Check sheet for the drawn part. Datum: minimum x, y, z corner. Units: mm. Round coordinates to 2 decimals unless told otherwise and drop trailing zeros. Write each loop counter-clockwise with the first axis right and the second up, starting at its lowest first coordinate (ties: lowest second). Pieces come first, ordered by that corner, then holes. Notation, with made-up numbers: (-25.75, 63) - (30.25, 63) arc R11 ccw to (30.25, 73) - close; hole circle Ø8 at (-28, 87). An arc over 180 degrees is marked (long way). Answer as a JSON object with one key per item and string values. Group by question number.
Item 1: Gauge pin test, flat end, axial feed: P1, Ø1.5, axis at y = 1.5, z = 1, coming from the -X side. Record the tip position at first contact, or that the pin passes through.
Item 2: Sectioned sample at A-A on x = 7. Record the boundary of the cut face in (y, z), plus the area to 3 significant figures.
Item 3: Release check for a two-part mould opening along Y. For the marked faces 1, 2 and 3 record: pulls with the +Y half, pulls with the -Y half, needs draft (parallel to the pull), parting line crosses it, or undercut.
Item 4: Sectioned sample at C-C on z = 9.25. Record the boundary of the cut face in (x, y), plus the area to 3 significant figures.
Item 5: Thickness scan on line 1 (Y direction, x = 7, z = 7.25); line 2 (Y direction, x = 4.75, z = 1.25). Record the ranges inside material, lowest first.
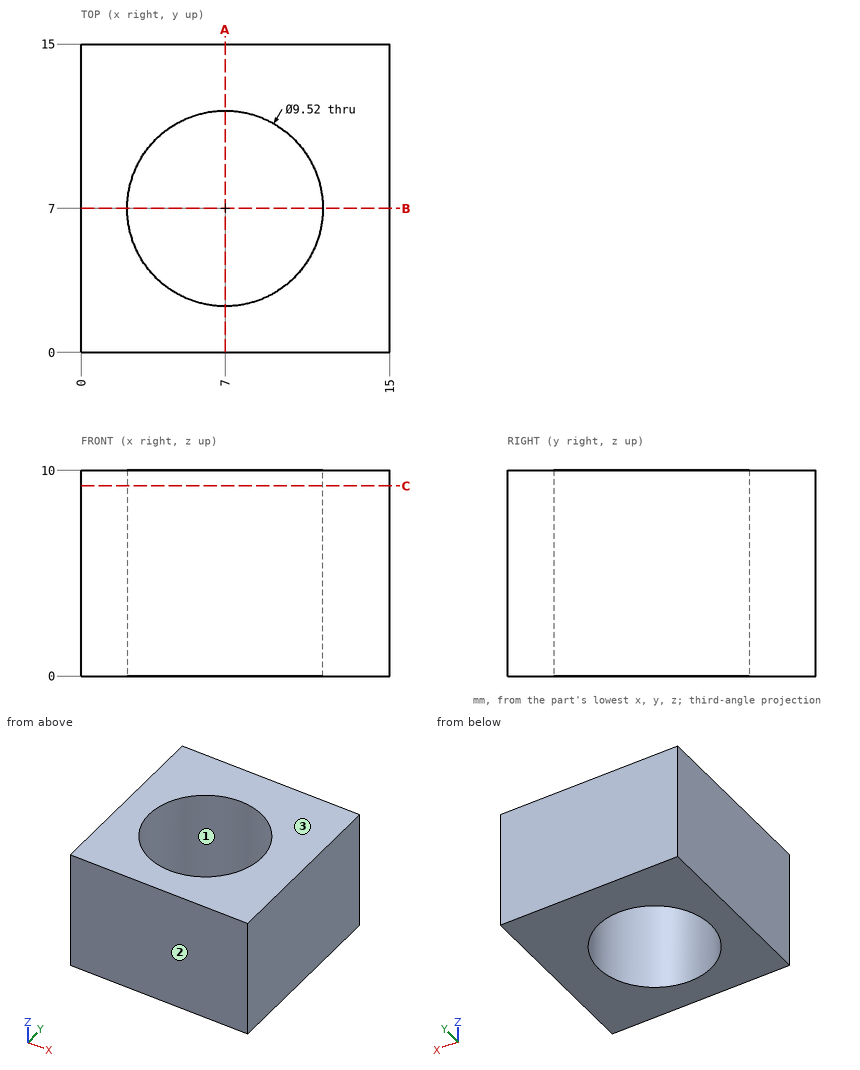
Completed:
{
 "1": {"P1": "x = 0"},
 "2": {"outline": "(0, 0) - (2.24, 0) - (2.24, 10) - (0, 10) - close; (11.76, 0) - (15, 0) - (15, 10) - (11.76, 10) - close", "area": "54.8 mm²"},
 "3": {"face 1": "undercut", "face 2": "pulls with the -Y half", "face 3": "needs draft"},
 "4": {"outline": "(0, 0) - (15, 0) - (15, 15) - (0, 15) - close; hole circle Ø9.52 at (7, 7)", "area": "154 mm²"},
 "5": {"line 1": "0 to 2.24, 11.76 to 15", "line 2": "0 to 2.81, 11.19 to 15"}
}
